from build123d import *

# Parameters (mm, degrees)
F0_R     = 20
F1_DEPTH = 5
F2_R     = 10.480538
F3_DEPTH = 5
F4_R     = 20
F5_DEPTH = 5
F7_DEPTH = 25


with BuildPart() as f1:
    # F0 (on Front) → F1 (new body)
    with BuildSketch(Plane.XZ):
        Circle(F0_R)
    extrude(amount=F1_DEPTH)

    # F2 (on face) → F3 (join)
    with BuildSketch(Plane.XZ.offset(5)):
        Circle(F2_R)
    extrude(amount=F3_DEPTH)

    # F4 (on face) → F5 (join)
    with BuildSketch(Plane.XZ.offset(10)):
        Circle(F4_R)
    extrude(amount=F5_DEPTH)

    # F6 (on face) → F7 (cut)
    with BuildSketch(Plane.XZ.offset(15)):
        Polygon((42.726062, 0), (-35.465427, 0), (-28.7633, -32.393619), (42.726062, -32.393619), align=None)
    extrude(amount=-F7_DEPTH, mode=Mode.SUBTRACT)


solid = f1.part
Could you check a few things on this model? Use its own coordinates, in mm. A direction names the side the tool comes from. Round coordinates to 2 decimals unless told otherwise and drop trailing zeros. Order: outer loops, then holes, each group sorted by start corner. A loop starts at its lowest first (then second) coordinate and runs counter-clockwise, first axis right, second up.
(1) Which directions (+Z, -Z, +X, -X, +Y, -Y) give clear straight access to the entire face, cutting with the end or side of a thin tool? Please do faces 4 (the flat face through (0, -10, 12)), 5 (the cylindrical face through (0, -2, 20)).
Response values:
face 4: +Z
face 5: +Z, +Y, -Y
(2) I'm going to push flat-ended pins straight in: pin 1 (1.5 mm diameter, centred on x = 15.5, z = 13, fed in from +Y); pin 2 (1.5 mm diameter, centred on x = 15, y = -10.5, fed in from +Z); pin 3 (5 mm diameter, centred on x = 11, y = -13.5, fed in from +Z). Where does each tip first touch, or does it pass through?
Response values:
pin 1: stops at y = 0
pin 2: stops at z = 14.03
pin 3: stops at z = 18.1
(3) Imagine slicing it at B-B (x = 0). Write out the boundary of the cut face in (y, z).
Response values:
outline: (-15, 0) - (0, 0) - (0, 20) - (-5, 20) - (-5, 10.48) - (-10, 10.48) - (-10, 20) - (-15, 20) - close
(4) Imagine slicing it at C-C (z = 13.75). Write out the boundary of the cut face in (x, y).
Response values:
outline: (-14.52, -15) - (14.52, -15) - (14.52, -10) - (-14.52, -10) - close; (-14.52, -5) - (14.52, -5) - (14.52, 0) - (-14.52, 0) - close
(5) If we mould it in two halves opening along Y, with no side actions, what happens to faces 1 (the cylindrical face through (0.23, -7.46, 10.48)), 2 (the flat face through (0, 0, 8)), 3 (the flat face through (0, -15, 8))? For each: released by +Y, released by -Y, zero draft, split by the parting line, or undercut.
Response values:
face 1: undercut
face 2: released by +Y
face 3: released by -Y
(6) Imagine slicing it at D-D (y = -9.5). Write out the boundary of the cut face in (x, z).
Response values:
outline: (-10.48, 0) - (10.48, 0) arc R10.48 ccw to start
(7) Please list where these lines run through material, in increasing order: line 1 along Y through (x, z) = (12, 11); line 2 along Z through (x, y) = (5, -13); line 3 along Z through (x, y) = (-7.5, -4).
Response values:
line 1: y = -15 to -10, -5 to 0
line 2: z = 0 to 19.36
line 3: z = 0 to 18.54
(8) Imagine slicing it at A-A (x = 16.5). Write out the boundary of the cut face in (y, z), plus the area to 3 significant figures.
Response values:
outline: (-15, 0) - (-10, 0) - (-10, 11.3) - (-15, 11.3) - close; (-5, 0) - (0, 0) - (0, 11.3) - (-5, 11.3) - close
area: 113 mm2
